```python
from build123d import *

# Parameters (mm, degrees)
SKETCH1_W             = 63.5
SKETCH1_H             = 63.5
BOSS_EXTRUDE1_DEPTH   = 704.85
SKETCH2_W             = 57.15
SKETCH2_H             = 57.15
CUT_EXTRUDE1_DEPTH    = 705.85
CUT_EXTRUDE2_REACH    = 65.5
SKETCH3_R             = 17.4625
SKETCH8_R             = 2.15265
CUT_EXTRUDE6_DEPTH    = 64.5
SKETCH10_R            = 2.15265
CUT_EXTRUDE7_DEPTH    = 64.5
CUT_EXTRUDE9_REACH    = 65.5
SKETCH13_R            = 16
SKETCH14_R            = 2.625
SKETCH14_R_2          = 16
CUT_EXTRUDE10_DEPTH   = 3.175
CUT_EXTRUDE11_START   = -3.175
CUT_EXTRUDE11_DEPTH   = 3.175
CUT_EXTRUDE13_REACH   = 65.5
SKETCH17_W            = 19.05
SKETCH17_H            = 25.4
SKETCH18_W            = 63.5
SKETCH18_H            = 63.5
CUT_EXTRUDE14_DEPTH   = 552.45
F_8_CLEARANCE_HOLE1_D = 4.3053
SKETCH21_R            = 2.15265
CUT_EXTRUDE15_DEPTH   = 6.35
SKETCH23_R            = 2.15265
CUT_EXTRUDE16_DEPTH   = 13.97


with BuildPart() as part:
    # Sketch1 → Boss-Extrude1 (new body)
    with BuildSketch(Plane(origin=(0, 0, 0), x_dir=(0, 0, -1), z_dir=(1, 0, 0))):
        Rectangle(SKETCH1_W, SKETCH1_H)
    extrude(amount=BOSS_EXTRUDE1_DEPTH)

    # Sketch2 → Cut-Extrude1 (cut, through all)
    with BuildSketch(Plane(origin=(704.85, 0, 0), x_dir=(0, 0, -1), z_dir=(1, 0, 0))):
        Rectangle(SKETCH2_W, SKETCH2_H)
    extrude(amount=-CUT_EXTRUDE1_DEPTH, mode=Mode.SUBTRACT)

    # Sketch3 → Cut-Extrude2 (cut, up to next)
    with BuildSketch(Plane.XY.offset(31.75), mode=Mode.PRIVATE) as cut_extrude2_sk1:
        with Locations((352.425, 0)):
            Circle(SKETCH3_R)
    cut_extrude2_tool1 = extrude(cut_extrude2_sk1.sketch, amount=-CUT_EXTRUDE2_REACH, mode=Mode.PRIVATE) & part.part
    add(cut_extrude2_tool1.solids().sort_by_distance((352.425, 0, 31.75))[0], mode=Mode.SUBTRACT)
    # Sketch3 → Cut-Extrude2 (cut, up to next)
    with BuildSketch(Plane.XY.offset(31.75), mode=Mode.PRIVATE) as cut_extrude2_sk2:
        with Locations((34.925, 0)):
            Circle(SKETCH3_R)
    cut_extrude2_tool2 = extrude(cut_extrude2_sk2.sketch, amount=-CUT_EXTRUDE2_REACH, mode=Mode.PRIVATE) & part.part
    add(cut_extrude2_tool2.solids().sort_by_distance((34.925, 0, 31.75))[0], mode=Mode.SUBTRACT)
    # Sketch3 → Cut-Extrude2 (cut, up to next)
    with BuildSketch(Plane.XY.offset(31.75), mode=Mode.PRIVATE) as cut_extrude2_sk3:
        with Locations((669.925, 0)):
            Circle(SKETCH3_R)
    cut_extrude2_tool3 = extrude(cut_extrude2_sk3.sketch, amount=-CUT_EXTRUDE2_REACH, mode=Mode.PRIVATE) & part.part
    add(cut_extrude2_tool3.solids().sort_by_distance((669.925, 0, 31.75))[0], mode=Mode.SUBTRACT)

    # Sketch8 → Cut-Extrude6 (cut, through all)
    with BuildSketch(Plane(origin=(0, 31.75, 0), x_dir=(1, 0, 0), z_dir=(0, 1, 0))):
        with Locations((466.725, 0)):
            Circle(SKETCH8_R)
        with Locations((123.825, 0)):
            Circle(SKETCH8_R)
        with Locations((581.025, 0)):
            Circle(SKETCH8_R)
        with Locations((238.125, 0)):
            Circle(SKETCH8_R)
    extrude(amount=-CUT_EXTRUDE6_DEPTH, mode=Mode.SUBTRACT)

    # Sketch10 → Cut-Extrude7 (cut, through all)
    with BuildSketch(Plane.XY.offset(31.75)):
        with Locations((225.425, 0)):
            Circle(SKETCH10_R)
        with Locations((568.325, 0)):
            Circle(SKETCH10_R)
        with Locations((136.525, 0)):
            Circle(SKETCH10_R)
        with Locations((479.425, 0)):
            Circle(SKETCH10_R)
    extrude(amount=-CUT_EXTRUDE7_DEPTH, mode=Mode.SUBTRACT)

    # Sketch13 → Cut-Extrude9 (cut, up to next)
    with BuildSketch(Plane(origin=(0, 0, -31.75), x_dir=(-1, 0, 0), z_dir=(0, 0, -1)), mode=Mode.PRIVATE) as cut_extrude9_sk1:
        with Locations((-352.425, 0)):
            Circle(SKETCH13_R)
    cut_extrude9_tool1 = extrude(cut_extrude9_sk1.sketch, amount=-CUT_EXTRUDE9_REACH, mode=Mode.PRIVATE) & part.part
    add(cut_extrude9_tool1.solids().sort_by_distance((352.425, 0, -31.75))[0], mode=Mode.SUBTRACT)
    # Sketch13 → Cut-Extrude9 (cut, up to next)
    with BuildSketch(Plane(origin=(0, 0, -31.75), x_dir=(-1, 0, 0), z_dir=(0, 0, -1)), mode=Mode.PRIVATE) as cut_extrude9_sk2:
        with Locations((-34.925, 0)):
            Circle(SKETCH13_R)
    cut_extrude9_tool2 = extrude(cut_extrude9_sk2.sketch, amount=-CUT_EXTRUDE9_REACH, mode=Mode.PRIVATE) & part.part
    add(cut_extrude9_tool2.solids().sort_by_distance((34.925, 0, -31.75))[0], mode=Mode.SUBTRACT)
    # Sketch13 → Cut-Extrude9 (cut, up to next)
    with BuildSketch(Plane(origin=(0, 0, -31.75), x_dir=(-1, 0, 0), z_dir=(0, 0, -1)), mode=Mode.PRIVATE) as cut_extrude9_sk3:
        with Locations((-669.925, 0)):
            Circle(SKETCH13_R)
    cut_extrude9_tool3 = extrude(cut_extrude9_sk3.sketch, amount=-CUT_EXTRUDE9_REACH, mode=Mode.PRIVATE) & part.part
    add(cut_extrude9_tool3.solids().sort_by_distance((669.925, 0, -31.75))[0], mode=Mode.SUBTRACT)

    # Sketch14 → Cut-Extrude10 (cut)
    with BuildSketch(Plane(origin=(0, 0, -31.75), x_dir=(-1, 0, 0), z_dir=(0, 0, -1))):
        with Locations((-655.782864376, 14.142135624)):
            Circle(SKETCH14_R)
        with Locations((-338.282864376, 14.142135624)):
            Circle(SKETCH14_R)
        with Locations((-20.782864376, 14.142135624)):
            Circle(SKETCH14_R)
        with Locations((-352.425, 0)):
            Circle(SKETCH14_R_2)
        with Locations((-34.925, 0)):
            Circle(SKETCH14_R_2)
        with Locations((-669.925, 0)):
            Circle(SKETCH14_R_2)
        with Locations((-338.282864376, -14.142135624)):
            Circle(SKETCH14_R)
        with Locations((-366.567135624, -14.142135624)):
            Circle(SKETCH14_R)
        with Locations((-366.567135624, 14.142135624)):
            Circle(SKETCH14_R)
        with Locations((-20.782864376, -14.142135624)):
            Circle(SKETCH14_R)
        with Locations((-49.067135624, -14.142135624)):
            Circle(SKETCH14_R)
        with Locations((-49.067135624, 14.142135624)):
            Circle(SKETCH14_R)
        with Locations((-655.782864376, -14.142135624)):
            Circle(SKETCH14_R)
        with Locations((-684.067135624, -14.142135624)):
            Circle(SKETCH14_R)
        with Locations((-684.067135624, 14.142135624)):
            Circle(SKETCH14_R)
    extrude(amount=-CUT_EXTRUDE10_DEPTH, mode=Mode.SUBTRACT)

    # Sketch15 → Cut-Extrude11 (cut)
    with BuildSketch(Plane.XY.offset(31.75).offset(CUT_EXTRUDE11_START)):
        with BuildLine():
            Line((364.710980323, -15.998290924), (362.776389114, -14.063699715))
            ThreePointArc((362.776389114, -14.063699715), (352.425, -17.4625), (342.073610886, -14.063699715))
            Line((342.073610886, -14.063699715), (340.139019677, -15.998290924))
            ThreePointArc((340.139019677, -15.998290924), (336.426709076, -15.998290924), (336.426709076, -12.285980323))
            Line((336.426709076, -12.285980323), (338.361300285, -10.351389114))
            ThreePointArc((338.361300285, -10.351389114), (334.9625, 0), (338.361300285, 10.351389114))
            Line((338.361300285, 10.351389114), (336.426709076, 12.285980323))
            ThreePointArc((336.426709076, 12.285980323), (336.426709076, 15.998290924), (340.139019677, 15.998290924))
            Line((340.139019677, 15.998290924), (342.073610886, 14.063699715))
            ThreePointArc((342.073610886, 14.063699715), (352.425, 17.4625), (362.776389114, 14.063699715))
            Line((362.776389114, 14.063699715), (364.710980323, 15.998290924))
            ThreePointArc((364.710980323, 15.998290924), (368.423290924, 15.998290924), (368.423290924, 12.285980323))
            Line((368.423290924, 12.285980323), (366.488699715, 10.351389114))
            ThreePointArc((366.488699715, 10.351389114), (369.8875, 0), (366.488699715, -10.351389114))
            Line((366.488699715, -10.351389114), (368.423290924, -12.285980323))
            ThreePointArc((368.423290924, -12.285980323), (368.423290924, -15.998290924), (364.710980323, -15.998290924))
        make_face()
        with BuildLine():
            Line((50.923290924, 12.285980323), (48.988699715, 10.351389114))
            ThreePointArc((48.988699715, 10.351389114), (52.3875, 0), (48.988699715, -10.351389114))
            Line((48.988699715, -10.351389114), (50.923290924, -12.285980323))
            ThreePointArc((50.923290924, -12.285980323), (50.923290924, -15.998290924), (47.210980323, -15.998290924))
            Line((47.210980323, -15.998290924), (45.276389114, -14.063699715))
            ThreePointArc((45.276389114, -14.063699715), (34.925, -17.4625), (24.573610886, -14.063699715))
            Line((24.573610886, -14.063699715), (22.639019677, -15.998290924))
            ThreePointArc((22.639019677, -15.998290924), (18.926709076, -15.998290924), (18.926709076, -12.285980323))
            Line((18.926709076, -12.285980323), (20.861300285, -10.351389114))
            ThreePointArc((20.861300285, -10.351389114), (17.4625, 0), (20.861300285, 10.351389114))
            Line((20.861300285, 10.351389114), (18.926709076, 12.285980323))
            ThreePointArc((18.926709076, 12.285980323), (18.926709076, 15.998290924), (22.639019677, 15.998290924))
            Line((22.639019677, 15.998290924), (24.573610886, 14.063699715))
            ThreePointArc((24.573610886, 14.063699715), (34.925, 17.4625), (45.276389114, 14.063699715))
            Line((45.276389114, 14.063699715), (47.210980323, 15.998290924))
            ThreePointArc((47.210980323, 15.998290924), (50.923290924, 15.998290924), (50.923290924, 12.285980323))
        make_face()
        with BuildLine():
            Line((685.923290924, 12.285980323), (683.988699715, 10.351389114))
            ThreePointArc((683.988699715, 10.351389114), (687.3875, 0), (683.988699715, -10.351389114))
            Line((683.988699715, -10.351389114), (685.923290924, -12.285980323))
            ThreePointArc((685.923290924, -12.285980323), (685.923290924, -15.998290924), (682.210980323, -15.998290924))
            Line((682.210980323, -15.998290924), (680.276389114, -14.063699715))
            ThreePointArc((680.276389114, -14.063699715), (669.925, -17.4625), (659.573610886, -14.063699715))
            Line((659.573610886, -14.063699715), (657.639019677, -15.998290924))
            ThreePointArc((657.639019677, -15.998290924), (653.926709076, -15.998290924), (653.926709076, -12.285980323))
            Line((653.926709076, -12.285980323), (655.861300285, -10.351389114))
            ThreePointArc((655.861300285, -10.351389114), (652.4625, 0), (655.861300285, 10.351389114))
            Line((655.861300285, 10.351389114), (653.926709076, 12.285980323))
            ThreePointArc((653.926709076, 12.285980323), (653.926709076, 15.998290924), (657.639019677, 15.998290924))
            Line((657.639019677, 15.998290924), (659.573610886, 14.063699715))
            ThreePointArc((659.573610886, 14.063699715), (669.925, 17.4625), (680.276389114, 14.063699715))
            Line((680.276389114, 14.063699715), (682.210980323, 15.998290924))
            ThreePointArc((682.210980323, 15.998290924), (685.923290924, 15.998290924), (685.923290924, 12.285980323))
        make_face()
    extrude(amount=CUT_EXTRUDE11_DEPTH, mode=Mode.SUBTRACT)

    # Sketch17 → Cut-Extrude13 (cut, up to next)
    with BuildSketch(Plane.XZ.offset(31.75), mode=Mode.PRIVATE) as cut_extrude13_sk1:
        with Locations((352.425, -12.7)):
            Rectangle(SKETCH17_W, SKETCH17_H)
    cut_extrude13_tool1 = extrude(cut_extrude13_sk1.sketch, amount=-CUT_EXTRUDE13_REACH, mode=Mode.PRIVATE) & part.part
    add(cut_extrude13_tool1.solids().sort_by_distance((352.425, -31.75, -12.7))[0], mode=Mode.SUBTRACT)

    # Sketch18 → Cut-Extrude14 (cut)
    with BuildSketch(Plane(origin=(704.85, 0, 0), x_dir=(0, 0, -1), z_dir=(1, 0, 0))):
        Rectangle(SKETCH18_W, SKETCH18_H)
    extrude(amount=-CUT_EXTRUDE14_DEPTH, mode=Mode.SUBTRACT)

    # #8 Clearance Hole1 (through all)
    with Locations(Plane(origin=(0, 31.75, 0), x_dir=(1, 0, 0), z_dir=(0, 1, 0))):
        with Locations((7.62, 19.05), (7.62, -12.7), (144.78, -12.7), (144.78, 19.05)):
            Hole(F_8_CLEARANCE_HOLE1_D / 2)

    # Sketch21 → Cut-Extrude15 (cut)
    with BuildSketch(Plane(origin=(0, -31.75, 0), x_dir=(-1, 0, 0), z_dir=(0, -1, 0))):
        with Locations((-18.4785, -12.85875)):
            Circle(SKETCH21_R)
    extrude(amount=-CUT_EXTRUDE15_DEPTH, mode=Mode.SUBTRACT)

    # Sketch23 → Cut-Extrude16 (cut)
    with BuildSketch(Plane(origin=(0, 28.575, 0), x_dir=(-1, 0, 0), z_dir=(0, -1, 0))):
        with Locations((-18.4785, -12.85875)):
            Circle(SKETCH23_R)
    extrude(amount=-CUT_EXTRUDE16_DEPTH, mode=Mode.SUBTRACT)


solid = part.part
```
Part model, mm, in its own coordinate system. A direction names the side the tool comes from. Round coordinates to 2 decimals unless told otherwise and drop trailing zeros. Loops run counter-clockwise (first coordinate to the right, second up) from the corner with the lowest first, then second, coordinate; pieces in that order, holes last.
1. Slice it at B-B (y = 0). Count the separate pieces of the cut face and the enclosed holes in it, and give its area (3 significant figures).
Solutions:
separate pieces: 6
enclosed holes: 0
area: 728 mm2
2. Drill centre lines: line 1 along Z through (x, y) = (7.62, 29.35); line 2 along X through (y, z) = (31, 12.7); line 3 along Y through (x, z) = (108.5, 0) (3 decimals). Where is each one in solid material? Low to high.
Solutions:
line 1: z = -31.75 to -21.2, -16.9 to 10.55, 14.85 to 31.75
line 2: x = 0 to 5.47, 9.77 to 16.33, 20.63 to 142.63, 146.93 to 152.4
line 3: y = -31.75 to -28.575, 28.575 to 31.75
3. Slice it at A-A (x = 107.5). Give the cut face in (y, z) (3 decimals), and give its area (3 significant figures).
Solutions:
outline: (-31.75, -31.75) - (31.75, -31.75) - (31.75, 31.75) - (-31.75, 31.75) - close; hole (-28.575, -28.575) - (28.575, -28.575) - (28.575, 28.575) - (-28.575, 28.575) - close
area: 766 mm2
4. Slice it at D-D (z = 0). Give the cut face in (x, y) (3 decimals), and give its area (3 significant figures).
Solutions:
outline: (0, -31.75) - (121.672, -31.75) - (121.672, -28.575) - (0, -28.575) - close; (0, 28.575) - (121.672, 28.575) - (121.672, 31.75) - (0, 31.75) - close; (125.978, -31.75) - (152.4, -31.75) - (152.4, -28.575) - (125.978, -28.575) - close; (125.978, 28.575) - (152.4, 28.575) - (152.4, 31.75) - (125.978, 31.75) - close
area: 940 mm2
5. Flat gauge pin, fed straight in: pin 1 (4 mm diameter, centred on x = 136.525, y = 0, fed in from -Z). Where does the tip first touch, or does it go through?
Solutions:
pin 1: passes through
6. Slice it at C-C (z = -19.05). Give the cut face in (x, y) (3 decimals).
Solutions:
outline: (0, -31.75) - (5.467, -31.75) - (5.467, -28.575) - (0, -28.575) - close; (0, 28.575) - (5.467, 28.575) - (5.467, 31.75) - (0, 31.75) - close; (9.773, -31.75) - (142.627, -31.75) - (142.627, -28.575) - (9.773, -28.575) - close; (9.773, 28.575) - (142.627, 28.575) - (142.627, 31.75) - (9.773, 31.75) - close; (146.933, -31.75) - (152.4, -31.75) - (152.4, -28.575) - (146.933, -28.575) - close; (146.933, 28.575) - (152.4, 28.575) - (152.4, 31.75) - (146.933, 31.75) - close
7. Two-plate mould, pull along X, no slides. Class faces 4 (the face through (77, 0, -28.575)), 5 (the face through (137.682, 1.815, 30.185)), 6 (the face through (152.4, -30, 3)): pulls with the +X half, pulls with the -X half, needs draft (parallel to the pull), parting line crosses it, or undercut.
Solutions:
face 4: needs draft
face 5: undercut
face 6: pulls with the +X half
8. 3-axis set-ups, long thin cutter, end or side, ignore diameter. For faces 1 (the face through (77, 0, 28.575)), 2 (the face through (75, 0, -31.75)), 3 (the face through (17.463, -0.155, 30.14)): which of +Z, -Z, +X, -X, +Y, -Y reach the whole face in a straight line?
Solutions:
face 1: +X, -X
face 2: -Z, +X, -X, +Y, -Y
face 3: +Z
